Read the model definition and answer for the solid it produces. Units are mm, in the model's axes. Give positions to 0.01 mm unless a question says otherwise; leave off trailing zeros. Order: outer loops, then holes, each group sorted by start corner. A loop starts at its lowest first (then second) coordinate and runs counter-clockwise, first axis right, second up.
```python
from build123d import *

# Parameters (mm, degrees)
F0_W     = 155
F0_H     = 105
F1_DEPTH = 25
F2_R     = 5
F3_SIZE  = 5


with BuildPart() as f1:
    # F0 (on Top) → F1 (new body)
    with BuildSketch(Plane.XY):
        Rectangle(F0_W, F0_H)
    extrude(amount=F1_DEPTH)

    # F2
    f2_edges = [f1.edges().sort_by_distance(p)[0] for p in [
        (-77.5, -52.5, 12.5),
        (-77.5, 52.5, 12.5),
        (77.5, -52.5, 12.5),
        (77.5, 52.5, 12.5),
    ]]
    fillet(f2_edges, radius=F2_R)

    # F3
    f3_edges = [f1.edges().sort_by_distance(p)[0] for p in [
        (0, 52.5, 25),
        (0, -52.5, 0),
    ]]
    chamfer(f3_edges, length=F3_SIZE)


solid = f1.part
```
1) Consider L1, parallel to Y at x = 30, z = 20.75; L2, parallel to Y at x = 59.5, z = 22; L3, parallel to X at y = 4, z = 23. Determine where each line is inside the solid, lowest interval first.
Final values:
L1: y = -51.75 to 51.75
L2: y = -50.5 to 50.5
L3: x = -74.5 to 74.5
2) The part is cut by section A-A on x = 12. Determine the outline of the cut face in (y, z).
Final values:
outline: (-52.5, 5) - (-47.5, 0) - (47.5, 0) - (52.5, 5) - (52.5, 20) - (47.5, 25) - (-47.5, 25) - (-52.5, 20) - close
3) For a pull along Z with two mould halves and no side action, classify faces 1 (the face through (75, -0.7, 2.5)), 2 (the face through (-76.07, -51, 12.6)), 3 (the face through (-74.312, 49.273, 22.465)) as released by +Z, released by -Z, zero draft, split by the parting line, or undercut.
Final values:
face 1: released by -Z
face 2: zero draft
face 3: released by +Z
